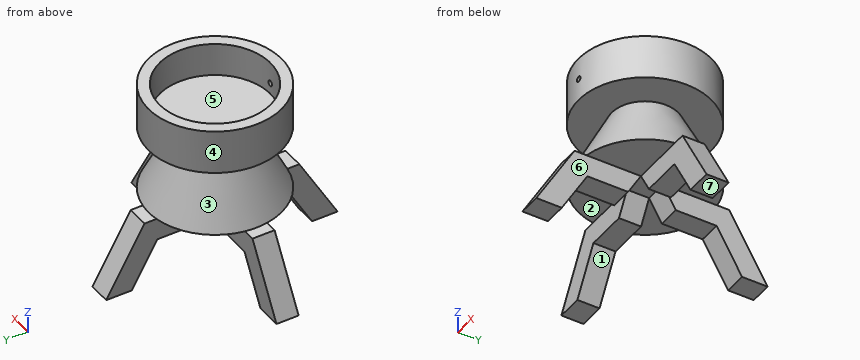
```python
from build123d import *

# Parameters (mm, degrees)
F2_DEPTH  = 25.4
F3_DEPTH  = 25.4
F4_R      = 152.4
F6_R      = 76.2
F8_R      = 152.4
F8_R_2    = 76.2
F9_DEPTH  = 101.6
F10_R     = 127
F11_DEPTH = 76.2
F13_DEPTH = 265.7891810245


with BuildPart() as f2:
    # F0 (on Front) → F2 (new body, symmetric)
    with BuildSketch(Plane.XZ):
        Polygon((177.8, 0), (25.4, 0), (54.7293936748, -50.8), (148.4706063252, -50.8), (177.8, -50.8), align=None)
        Polygon((207.1293936748, -50.8), (177.8, 0), (177.8, -50.8), align=None)
        Polygon((177.8, -50.8), (148.4706063252, -50.8), (177.8, -101.6), align=None)
        Polygon((207.1293936748, -50.8), (177.8, -50.8), (177.8, -101.6), (207.1293936748, -152.4), (265.7881810245, -152.4), align=None)
    extrude(amount=F2_DEPTH, both=True)



with BuildPart() as f2b:
    # F0 (on Front) → F2, piece 2 (new body, symmetric)
    with BuildSketch(Plane.XZ):
        Polygon((-54.7293936748, -50.8), (-25.4, 0), (-177.8, 0), (-207.1293936748, -50.8), (-148.4706063252, -50.8), align=None)
        Polygon((-207.1293936748, -152.4), (-148.4706063252, -50.8), (-207.1293936748, -50.8), (-265.7881810245, -152.4), align=None)
    extrude(amount=F2_DEPTH, both=True)


with BuildPart() as f2_1:
    add(f2.part)

    add(f2b.part)  # F3 merges F2b
    # F1 (on Right) → F3 (join, symmetric)
    with BuildSketch(Plane.YZ):
        Polygon((177.8, 0), (25.4, 0), (54.7293936748, -50.8), (148.4706063252, -50.8), (177.8, -50.8), align=None)
        Polygon((-54.7293936748, -50.8), (-25.4, 0), (-177.8, 0), (-207.1293936748, -50.8), (-148.4706063252, -50.8), align=None)
        Polygon((207.1293936748, -50.8), (177.8, 0), (177.8, -50.8), align=None)
        Polygon((177.8, -50.8), (148.4706063252, -50.8), (177.8, -101.6), align=None)
        Polygon((207.1293936748, -50.8), (177.8, -50.8), (177.8, -101.6), (207.1293936748, -152.4), (222.5192777686, -152.4), (265.7881810245, -152.4), align=None)
        Polygon((-207.1293936748, -152.4), (-148.4706063252, -50.8), (-207.1293936748, -50.8), (-265.7881810245, -152.4), align=None)
    extrude(amount=F3_DEPTH, both=True)

    # F4 (on Top) → F7 section 0
    with BuildSketch(Plane.XY):
        Circle(F4_R)
    # F6 (on offset) → F7 section 1
    with BuildSketch(Plane.XY.offset(152.4)):
        Circle(F6_R)
    loft()

    # F8 (on face) → F9 (join)
    with BuildSketch(Plane.XY.offset(152.4)):
        Circle(F8_R)
        Circle(F8_R_2, mode=Mode.SUBTRACT)
        Circle(F8_R_2)
    extrude(amount=F9_DEPTH)

    # F10 (on face) → F11 (cut)
    with BuildSketch(Plane.XY.offset(254)):
        Circle(F10_R)
    extrude(amount=-F11_DEPTH, mode=Mode.SUBTRACT)

    # F12 (on Front) → F13 (cut, through all)
    with BuildSketch(Plane.XZ):
        with BuildLine():
            ThreePointArc((0, 196.85), (4.4901280605, 198.7098719395), (6.35, 203.2))
            ThreePointArc((6.35, 203.2), (-4.4901280605, 207.6901280605), (0, 196.85))
        make_face()
    extrude(amount=F13_DEPTH, mode=Mode.SUBTRACT)


solid = f2_1.part
```
Here's how the part is built. I have some questions about the finished solid (model axes, mm). Face numbers are marked on the shaded views. A direction names the side the tool comes from. Round coordinates to 2 decimals unless told otherwise and drop trailing zeros. Order: outer loops, then holes, each group sorted by start corner. A loop starts at its lowest first (then second) coordinate and runs counter-clockwise, first axis right, second up. Notation, with made-up numbers: M 8.25,30.5 L 22.25,30.5 A27 ccw 22.25,69.5 Z; hole C -35,19 d5. An arc over 180 degrees is marked long. Answer in a Markdown table with one row per item.
Item 1: Thinking about a two-plate mould opening in X: for the marked faces 4, 5, 6 and 7, which applies, +X half, -X half, draft (parallel to the pull), parting line (faces both ways), or undercut?
A:
| item | result |
|---|---|
| face 4 | parting line |
| face 5 | undercut |
| face 6 | +X half |
| face 7 | draft |
Item 2: For the marked faces 1, 2 and 3, which set-ups out of +Z, -Z, +X, -X, +Y, -Y let a thin tool reach every point of the face, with its end or its side?
A:
| item | result |
|---|---|
| face 1 | -Z, +Y, -Y |
| face 2 | -Z, -X, -Y |
| face 3 | none |
Item 3: Imagine slicing it at B-B, the plane x = -187.5. Write out the boundary of the cut face in (y, z).
A:
| item | result |
|---|---|
| outline | M -25.4,-118.4 L 25.4,-118.4 L 25.4,-16.8 L -25.4,-16.8 Z |
Item 4: Imagine slicing it at A-A, the plane z = 70. Write out the boundary of the cut face in (x, y), and give its area (3 significant figures).
A:
| item | result |
|---|---|
| outline | C 0,0 d234.8 |
| area | 43,300 mm2 |
Item 5: If I drill on L1, parallel to Y at x = 0, z = 195.5; L2, parallel to Z at x = 0, y = -141; L3, parallel to Z at x = 0, y = -138.5, over which ranges is the centre line in solid material (lowest first)? Write a range as from..to.
A:
| item | result |
|---|---|
| L1 | y = -152.4..-127, 127..152.4 |
| L2 | z = -50.8..22.8, 152.4..196.85, 209.55..254 |
| L3 | z = -50.8..27.8, 152.4..196.85, 209.55..254 |
Item 6: I'm going to push flat-ended pins straight in: pin 1 (4 mm diameter, centred on x = 89, y = -39, fed in from -Z); pin 2 (8.5 mm diameter, centred on x = 161, y = 7, fed in from +Z); pin 3 (1.5 mm diameter, centred on x = -40, z = 163, fed in from +Y). Where does each tip first touch, or does it pass through?
A:
| item | result |
|---|---|
| pin 1 | stops at z = 0 |
| pin 2 | stops at z = 0 |
| pin 3 | stops at y = 147.26 |
